Work out the finished part from the listing and answer in its coordinate system (mm). Give positions to 0.01 mm unless a question says otherwise; leave off trailing zeros. Write each loop counter-clockwise with the first axis right and the second up, starting at its lowest first coordinate (ties: lowest second). Pieces come first, ordered by that corner, then holes.
1) Given pin 1 Ø11 at (x, z) = (-59, 73) entering from +Y; pin 2 Ø12 at (y, z) = (-4.5, 49.5) entering from +X; pin 3 Ø4 at (x, z) = (-288, 71.5) entering from -Y, each flat-ended and moving along its own axis, determine where each tip first touches the part or whether it passes through.
2) Find section B-B (z = 47.5). Determine the outline of the cut face in (x, y), plus the area to 3 significant figures.
3) Straight lines are drawn through the part: probe 1 along X at (y, z) = (-10.5, 57); probe 2 along Y at (x, z) = (-349.5, 72.5); probe 3 along Z at (x, y) = (-265, -13). For each, find the intervals that lie inside material, in ascending order.
4) Find section A-A (x = 403). Determine the outline of the cut face in (y, z).
```python
from build123d import *

# Parameters (mm, degrees)
F1_W     = 40
F1_H     = 33
F3_DEPTH = 600
F2_W     = 80
F2_H     = 100
F4_DEPTH = 25
F5_W     = 1200
F5_H     = 50
F6_DEPTH = 1235


# Not quite as in the source:
# - an extrude ends at something that could not be found from the text; its depth is read off the source's solid


with BuildPart() as f3:
    # F1 (on Right) → F3 (new body, symmetric)
    with BuildSketch(Plane.YZ):
        Polygon((20, 33), (20, 63), (17, 66), (12, 66), (12, 80), (4, 80), (4, 66), (-4, 66), (-4, 80), (-12, 80), (-12, 66), (-17, 66), (-20, 63), (-20, 33), align=None)
        with Locations((0, 16.5)):
            Rectangle(F1_W, F1_H)
        with Locations((0, -16.5)):
            Rectangle(F1_W, F1_H)
    extrude(amount=F3_DEPTH, both=True)

    # F2 (on Front) → F4 (cut, symmetric)
    with BuildSketch(Plane.XZ):
        with Locations((600, 83)):
            Rectangle(F2_W, F2_H)
        with Locations((600, -83)):
            Rectangle(F2_W, F2_H)
    extrude(amount=F4_DEPTH, both=True, mode=Mode.SUBTRACT)

    # F5 (on face) → F6 (cut, through all)
    with BuildSketch(Plane.XZ.offset(20)):
        with Locations((0, -58)):
            Rectangle(F5_W, F5_H)
    extrude(amount=-F6_DEPTH, mode=Mode.SUBTRACT)


solid = f3.part
```
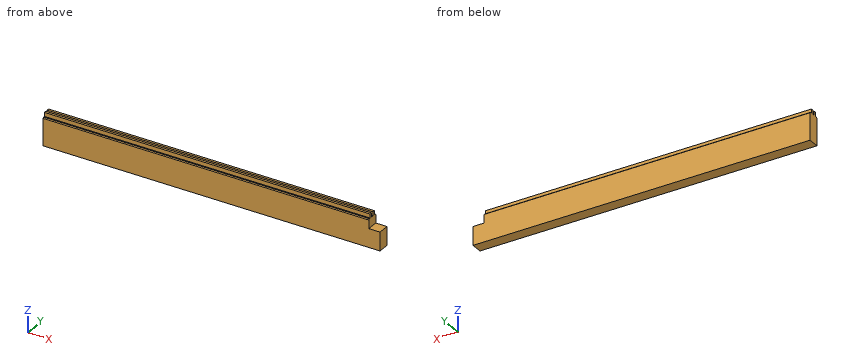
Results:
1. pin 1: stops at y = 12
1. pin 2: stops at x = 560
1. pin 3: stops at y = -12
2. outline: (-600, -20) - (560, -20) - (560, 20) - (-600, 20) - close
2. area: 46,400 mm2
3. probe 1: x = -600 to 560
3. probe 2: y = -12 to -4, 4 to 12
3. probe 3: z = -33 to 66
4. outline: (-20, -33) - (20, -33) - (20, 63) - (17, 66) - (12, 66) - (12, 80) - (4, 80) - (4, 66) - (-4, 66) - (-4, 80) - (-12, 80) - (-12, 66) - (-17, 66) - (-20, 63) - close
